Design review of the part built by this model. Coordinates are the model's own, in mm. Face numbers are marked on the shaded views. Coordinates: 2 decimals unless noted, no trailing zeros. Loops run counter-clockwise (first coordinate to the right, second up) from the corner with the lowest first, then second, coordinate; pieces in that order, holes last. Notation, with made-up numbers: (15, 23.25) -> (43, 23.25) arc R25 cw to (43, 43.25) -> close; hole circle Ø11 at (2.5, -12.75). An arc over 180 degrees is marked (long way). Use a Markdown table: item, result. Add a question column.
Q1. Take a section at A-A on z = 5. Write out the cut boundary in (x, y).
Q2. Draft analysis for pull direction Z (two halves, no side actions). For the marked faces 1, 2, 3 and 4, state which applies: pulls with the +Z half, pulls with the -Z half, needs draft (parallel to the pull), parting line crosses it, or undercut.
Q3. Clearance check with flat-ended pins moving along their axes: pin 1 Ø5 at (x, z) = (4.5, 24.5) entering from -Y; pin 2 Ø2 at (x, y) = (-4, -4) entering from +Z; pin 3 Ø10 at (x, z) = (-6, 25.5) entering from -Y. State where each tip first meets the part, or that it passes through.
Q4. For probe 1 along Z at (x, y) = (-0.5, -5.5); probe 2 along Z at (x, y) = (6, 6); probe 3 along Z at (x, y) = (1.5, -2.25), list the stretches that pass through material, from the lowest coordinate up.
Q5. Take a section at B-B on x = 0. Write out the cut boundary in (y, z).
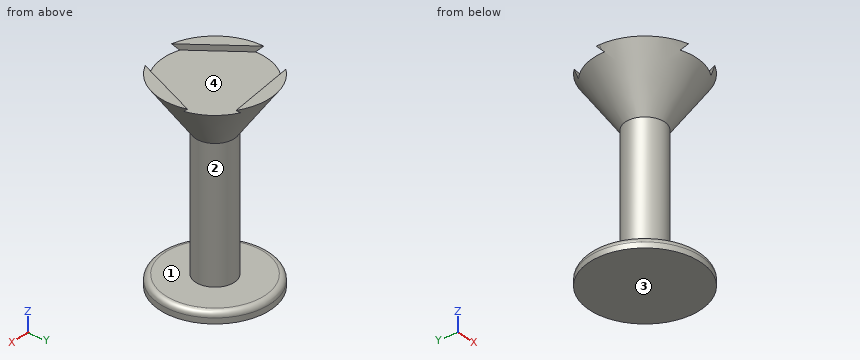
from build123d import *

# Parameters (mm, degrees)
F0_R     = 10
F1_DEPTH = 2
F3_R     = 1
F6_DEPTH = 1


with BuildPart() as f1:
    # F0 (on Top) → F1 (new body)
    with BuildSketch(Plane.XY):
        Circle(F0_R)
    extrude(amount=F1_DEPTH)

    # F3
    f3_edges = [f1.edges().sort_by_distance(p)[0] for p in [
        (-10, 0, 2),
    ]]
    fillet(f3_edges, radius=F3_R)

    # F2 (on Front) → F4 (revolve)
    with BuildSketch(Plane.XZ):
        Polygon((0, 35), (-10, 35), (-3.5, 25.7257949561), (-3.5, 2), (0, 2), align=None)
    revolve(axis=Axis((0, 0, 18.5), (0, 0, -1)))

    # F5 (on face) → F6 (cut)
    with BuildSketch(Plane.XY.offset(35)):
        Polygon((1.8076821121, -15.1926172437), (12.253351427, 9.1618072529), (-14.0610335391, 6.0308099908), align=None)
    extrude(amount=-F6_DEPTH, mode=Mode.SUBTRACT)


solid = f1.part
Answer list:
| question | item | result |
|---|---|---|
| 1 | outline | circle Ø7 at (0, 0) |
| 2 | face 1 | undercut |
| 2 | face 2 | undercut |
| 2 | face 3 | pulls with the -Z half |
| 2 | face 4 | pulls with the +Z half |
| 3 | pin 1 | y = -2.87 |
| 3 | pin 2 | z = 34 |
| 3 | pin 3 | y = -5.37 |
| 4 | probe 1 | 0 to 2, 28.61 to 34 |
| 4 | probe 2 | 0 to 2, 32.84 to 34 |
| 4 | probe 3 | 0 to 34 |
| 5 | outline | (-10, 0) -> (10, 0) -> (10, 1) arc R1 ccw to (9, 2) -> (3.5, 2) -> (3.5, 25.73) -> (10, 35) -> (7.7, 35) -> (7.7, 34) -> (-9.3, 34) -> (-3.5, 25.73) -> (-3.5, 2) -> (-9, 2) arc R1 ccw to (-10, 1) -> close |
